Verification items for the finished model (mm, model axes). A direction names the side the tool comes from. Give positions to 0.01 mm unless a question says otherwise; leave off trailing zeros. Order: outer loops, then holes, each group sorted by start corner. A loop starts at its lowest first (then second) coordinate and runs counter-clockwise, first axis right, second up. Notation, with made-up numbers: (-9.5, 9.5) -> (46.5, 9.5) arc R19 ccw to (46.5, 18.5) -> close; hole circle Ø5 at (33, 21.5). An arc over 180 degrees is marked (long way). One line per question, with ' | ' between items. Start each with the question number.
Q1. Material ranges on probe 1 along Y at (x, z) = (14.5, 0.5); probe 2 along Y at (x, z) = (18, 0.45), recorded low to high. Write a range as [from, to].
Q2. Section check B-B on x = 2. Record the cut outline in (y, z).
Q3. Section check A-A on z = 1.05. Record the cut outline in (x, y).
Q4. Access from +Z, -Z, +X, -X, +Y, -Y to the whole of each face (thin tool, end or side, straight path). Record for faces 5 (the flat face through (-15, -34, 1)), 6 (the flat face through (3, -34, 1)), 7 (the flat face through (11, -30, 1)), 8 (the flat face through (-13, -38, 1)).
Q5. Go/stop test with flat-tipped pins: pin 1 (1 mm diameter, centred on y = -32.5, z = 1, fed in from -X); pin 2 (1 mm diameter, centred on y = -33.5, z = 1.5, fed in from +X). Record where each tip stops, or that it passes through.
Q6. Mould release check, pull along X, two halves, no side actions. Record for faces 1 (the cylindrical face through (-18.859, -28.797, 1.014)), 2 (the flat face through (5, -38, 1)), 3 (the flat face through (7, -34, 1)), 4 (the flat face through (-11, -34, 1)): released by +X, released by -X, zero draft, split by the parting line, or undercut.
from build123d import *

# Parameters (mm, degrees)
SKETCH_1_W      = 40
SKETCH_1_H      = 60
SKETCH_1_W_2    = 4
SKETCH_1_H_2    = 8
EXTRUDE_1_DEPTH = 2
FILLET_1_R      = 4


with BuildPart() as part:
    # 草图1 → 凸台-拉伸1 (new body)
    with BuildSketch(Plane.XY):
        Rectangle(SKETCH_1_W, SKETCH_1_H)
        with Locations((-13, -34)):
            Rectangle(SKETCH_1_W_2, SKETCH_1_H_2)
        with Locations((5, -34)):
            Rectangle(SKETCH_1_W_2, SKETCH_1_H_2)
    extrude(amount=EXTRUDE_1_DEPTH)

    # 圆角1
    fillet_1_edges = [part.edges().sort_by_distance(p)[0] for p in [
        (20, -30, 1),
        (-20, -30, 1),
        (-20, 30, 1),
        (20, 30, 1),
    ]]
    fillet(fillet_1_edges, radius=FILLET_1_R)


solid = part.part
Filled in:
1) probe 1: [-30, 30] | probe 2: [-29.46, 29.46]
2) outline: (-30, 0) -> (30, 0) -> (30, 2) -> (-30, 2) -> close
3) outline: (-20, -26) arc R4 ccw to (-16, -30) -> (-15, -30) -> (-15, -38) -> (-11, -38) -> (-11, -30) -> (3, -30) -> (3, -38) -> (7, -38) -> (7, -30) -> (16, -30) arc R4 ccw to (20, -26) -> (20, 26) arc R4 ccw to (16, 30) -> (-16, 30) arc R4 ccw to (-20, 26) -> close
4) face 5: +Z, -Z, -X, -Y | face 6: +Z, -Z, -Y | face 7: +Z, -Z, +X, -Y | face 8: +Z, -Z, +X, -X, -Y
5) pin 1: x = -15 | pin 2: x = 7
6) face 1: released by -X | face 2: zero draft | face 3: released by +X | face 4: undercut
